Part model, mm, in its own coordinate system. A direction names the side the tool comes from. Round coordinates to 2 decimals unless told otherwise and drop trailing zeros. Write each loop counter-clockwise with the first axis right and the second up, starting at its lowest first coordinate (ties: lowest second). Pieces come first, ordered by that corner, then holes. Notation, with made-up numbers: M -24.5,38.25 L 17.5,38.25 A10 cw 17.5,45.25 Z; hole C -17,54.25 d7. An arc over 180 degrees is marked long. One line per question, with ' | ' between items. Start each with the question number.
1) Wall check: probe 1 along Z at (x, y) = (60.5, 0.7); probe 2 along Z at (x, y) = (32, 5.05); probe 3 along Z at (x, y) = (85, 3.75). Give the ranges that are in metal, low to high. Write a range as [from, to].
2) Tool access for faces 5 (the face through (31, 1, -52.5)), 6 (the face through (0, 3, -14)), 7 (the face through (83, 3, -30)), 8 (the face through (7, 3, -28.5)), 9 (the face through (48, 4, -5)): list every direction of +Z, -Z, +X, -X, +Y, -Y with a clear straight run to the whole face (end or side of a thin tool).
3) Saw through at C-C (z = -30). List the corners of the cut face in (x, y).
4) Drop flat-ended pins along their axis: pin 1 Ø5 at (x, z) = (62, -14) entering from -Y; pin 2 Ø1 at (y, z) = (2.5, -25) entering from -X; pin 3 Ø1 at (x, z) = (77, -30.5) entering from +Y; pin 4 Ø0.6 at (y, z) = (1, -27.5) entering from +X. Give the stop position or say it passes through.
5) Mould opens along Z. For faces 1 (the face through (36, 0, -30)), 2 (the face through (7, 4, -23.5)), 3 (the face through (64, 1, -23)), 4 (the face through (1, 3, -58)) say: pulls with the +Z half, pulls with the -Z half, needs draft (parallel to the pull), parting line crosses it, or undercut.
6) Saw through at A-A (z = -50). List the corners of the cut face in (x, y), plus the area to 3 significant figures.
7) Saw through at B-B (x = 35). List the corners of the cut face in (y, z), plus the area to 3 significant figures.
```python
from build123d import *

# Parameters (mm, degrees)
SKETCH1_W           = 95
SKETCH1_H           = 60
BOSS_EXTRUDE1_DEPTH = 6
SKETCH6_R           = 3.5
SKETCH6_R_2         = 1.5
CUT_EXTRUDE3_DEPTH  = 113.521109131
CUT_EXTRUDE1_DEPTH  = 4
CUT_EXTRUDE2_DEPTH  = 113.521109131
FILLET3_R           = 1.5
SKETCH7_W           = 8.5
SKETCH7_H           = 3
SKETCH7_H_2         = 7
CUT_EXTRUDE4_DEPTH  = 113.521109131
FILLET4_R           = 5
FILLET5_R           = 1.5


with BuildPart() as part:
    # Sketch1 → Boss-Extrude1 (new body)
    with BuildSketch(Plane(origin=(0, 0, 0), x_dir=(1, 0, 0), z_dir=(0, 1, 0))):
        with Locations((47.5, 30)):
            Rectangle(SKETCH1_W, SKETCH1_H)
    extrude(amount=BOSS_EXTRUDE1_DEPTH)

    # Sketch6 → Cut-Extrude3 (cut, through all)
    with BuildSketch(Plane.XZ):
        with Locations(Location((86.5, -30, 0), (0, 0, 270))):
            Circle(SKETCH6_R)
        with Locations(Location((8.5, -30, 0), (0, 0, 270))):
            Circle(SKETCH6_R_2)
    extrude(amount=-CUT_EXTRUDE3_DEPTH, mode=Mode.SUBTRACT)

    # Sketch2 → Cut-Extrude1 (cut)
    with BuildSketch(Plane(origin=(0, 6, 0), x_dir=(-1, 0, 0), z_dir=(0, 1, 0))):
        with BuildLine():
            Line((-8.5, -36.5), (-5, -36.5))
            Line((-5, -36.5), (-5, -55))
            Line((-5, -55), (-90, -55))
            Line((-90, -55), (-90, -38.5))
            Line((-90, -38.5), (-86.5, -38.5))
            ThreePointArc((-86.5, -38.5), (-78, -30), (-86.5, -21.5))
            Line((-86.5, -21.5), (-90, -21.5))
            Line((-90, -21.5), (-90, -5))
            Line((-90, -5), (-5, -5))
            Line((-5, -5), (-5, -23.5))
            Line((-5, -23.5), (-8.5, -23.5))
            ThreePointArc((-8.5, -23.5), (-15, -30), (-8.5, -36.5))
        make_face()
    extrude(amount=-CUT_EXTRUDE1_DEPTH, mode=Mode.SUBTRACT)

    # Sketch5 → Cut-Extrude2 (cut, through all)
    with BuildSketch(Plane.XZ):
        Polygon((46.75, -37), (46.75, -23), (16.5, -23), (16.5, -21.5), (46.75, -21.5), (46.75, -7.5), (16.5, -7.5), (16.5, -6), (47.5, -6), (78.5, -6), (78.5, -7.5), (48.25, -7.5), (48.25, -21.5), (78.5, -21.5), (78.5, -23), (48.25, -23), (48.25, -37), (78.5, -37), (78.5, -38.5), (48.25, -38.5), (48.25, -52.5), (78.5, -52.5), (78.5, -54), (47.5, -54), (16.5, -54), (16.5, -52.5), (46.75, -52.5), (46.75, -38.5), (16.5, -38.5), (16.5, -37), align=None)
    extrude(amount=-CUT_EXTRUDE2_DEPTH, mode=Mode.SUBTRACT)

    # Fillet3
    fillet3_edges = [part.edges().sort_by_distance(p)[0] for p in [
        (90, 4, -55),
    ]]
    fillet(fillet3_edges, radius=FILLET3_R)

    # Sketch7 → Cut-Extrude4 (cut, through all)
    with BuildSketch(Plane(origin=(0, 6, 0), x_dir=(-1, 0, 0), z_dir=(0, 1, 0))):
        with Locations((-4.25, -30)):
            Rectangle(SKETCH7_W, SKETCH7_H)
        with Locations((-90.75, -30)):
            Rectangle(SKETCH7_W, SKETCH7_H_2)
    extrude(amount=-CUT_EXTRUDE4_DEPTH, mode=Mode.SUBTRACT)

    # Fillet4
    fillet4_edges = [part.edges().sort_by_distance(p)[0] for p in [
        (0, 3, -28.5),
        (0, 3, -31.5),
        (95, 3, -33.5),
        (95, 3, -26.5),
        (0, 3, -60),
        (95, 3, -60),
        (95, 3, 0),
        (0, 3, 0),
    ]]
    fillet(fillet4_edges, radius=FILLET4_R)

    # Fillet5
    fillet5_edges = [part.edges().sort_by_distance(p)[0] for p in [
        (5, 4, -5),
        (5, 4, -23.5),
        (5, 4, -36.5),
        (5, 4, -55),
        (90, 4, -38.5),
        (90, 4, -21.5),
        (90, 4, -5),
    ]]
    fillet(fillet5_edges, radius=FILLET5_R)


solid = part.part
```
Answer key:
1) probe 1: z = [-60, -54], [-52.5, -38.5], [-37, -23], [-21.5, -7.5], [-6, 0] | probe 2: z = [-60, -55], [-5, 0] | probe 3: z = [-60, -55], [-38.37, -33.16], [-26.84, -21.63], [-5, 0]
2) face 5: +Y, -Y | face 6: +Z, -Z, -X, +Y, -Y | face 7: +X, +Y, -Y | face 8: -X, +Y, -Y | face 9: +Y
3) outline: M 10,0 L 46.75,0 L 46.75,2 L 15,2 L 15,6 L 10,6 Z; M 48.25,0 L 83,0 L 83,6 L 78,6 L 78,2 L 48.25,2 Z
4) pin 1: stops at y = 0 | pin 2: stops at x = 0.1 | pin 3: stops at y = 2 | pin 4: stops at x = 84.4
5) face 1: needs draft | face 2: undercut | face 3: undercut | face 4: pulls with the -Z half
6) outline: M 0,0 L 46.75,0 L 46.75,2 L 5,2 L 5,6 L 0,6 Z; M 48.25,0 L 95,0 L 95,6 L 90,6 L 90,2 L 48.25,2 Z | area: 227 mm2
7) outline: M 0,-60 L 6,-60 L 6,-55 L 2,-55 L 2,-54 L 0,-54 Z; M 0,-52.5 L 2,-52.5 L 2,-38.5 L 0,-38.5 Z; M 0,-37 L 2,-37 L 2,-23 L 0,-23 Z; M 0,-21.5 L 2,-21.5 L 2,-7.5 L 0,-7.5 Z; M 0,-6 L 2,-6 L 2,-5 L 6,-5 L 6,0 L 0,0 Z | area: 148 mm2
